Source: CAD feature listing. Evaluate the final solid. Frame: model axes, mm. A direction names the side the tool comes from. Give positions to 0.01 mm unless a question says otherwise; leave off trailing zeros. Order: outer loops, then holes, each group sorted by start corner. A loop starts at its lowest first (then second) coordinate and runs counter-clockwise, first axis right, second up. Notation, with made-up numbers: M -9,48 L 14,48 A20 ccw 14,60 Z; hole C 59.5,38 d6. An arc over 180 degrees is marked long. Use CSV: the item, a comma, the result in double quotes. Start each with the question number.
Item 1: Access query for faces 1 (the face through (0, 182, 23)), 2 (the face through (83.546, 357.97, 54.214)), 3 (the face through (152, 1.588, 38)). Directions: +Z, -Z, +X, -X, +Y, -Y. A direction counts if a zero-diameter tool reaches every point of the face in a straight line with its end or side. Return the directions, or none.
Item 2: First-contact query: pin 1 (6 mm diameter, centred on x = 40, y = 154.5, fed in from -Z); pin 2 (6 mm diameter, centred on x = 214, y = 196.5, fed in from +Z); pin 3 (1.3 mm diameter, centred on x = -2, y = 147, fed in from -Z); pin 4 (5 mm diameter, centred on y = 26.99, z = 52.39, fed in from -X). Flat tips, straight axial feed; report the tip coordinate or a pass-through.
Item 3: Section query A-A on y = 152.4. Return loops of the section in (x, z) (1 decimal).
Item 4: Pull-direction query (Z, two-part tool) for faces 4 (the face through (154, 358.775, 38)), 5 (the face through (152, 182, 0)), 6 (the face through (307.17, 141.382, 20.497)); classes: +Z half, -Z half, draft (parallel to the pull), parting line (faces both ways), or undercut.
Item 5: Ray query, probe 1 along X at (y, z) = (108, 60.5) (1 decimal); probe 2 along Y at (x, z) = (225.5, 13.5) (1 decimal); probe 3 along X at (y, z) = (183, 55) (1 decimal). Return the intervals inside material, ascending. Write a range as from..to.
Item 6: Section query C-C on x = 162.5. Return loops of the section in (y, z) (1 decimal), and give its area (3 significant figures).
Item 7: Section query D-D on x = 88.9. Count the separate pieces of the cut face and the enclosed holes in it, and give its area (3 significant figures).
Item 8: Section query B-B on z = 19.05. Return loops of the section in (x, y) (1 decimal), and give its area (3 significant figures).
Autodesk Inventor part; units mm, degrees
ref_plane "YZ Plane" through (0, 0, 0) normal (1, 0, 0) x (0, 1, 0)
ref_plane "XZ Plane" through (0, 0, 0) normal (0, 1, 0) x (-1, 0, 0)
ref_plane "XY Plane" through (0, 0, 0) normal (0, 0, 1) x (1, 0, 0)
sketch "Sketch1" plane through (0, 0, 0) normal (0, 0, 1) x (1, 0, 0)
  line L0 (0, 0) -> (307.975, 0)
  line L1 (307.975, 0) -> (307.975, 358.775)
  line L2 (307.975, 358.775) -> (0, 358.775)
  line L3 (0, 358.775) -> (0, 0)
  dimension "d0" = 307.975
  dimension "d1" = 358.775
extrude "Extrusion1" add sketch "Sketch1" along normal blind 76.2
shell "Shell1" thickness 1.5875 removed faces 1 at (205.3167, 119.5917, 76.2)
sketch "Sketch2" plane through (0, 358.775, 0) normal (0, 1, 0) x (1, 0, 0)
  line L0 (0, -76.2) -> (0, -60.325) construction
  line L1 (0, -60.325) -> (-3.175, -60.325) construction
  arc A0 (-2.3813, -58.7375) -> (-0.7938, -60.325) centre (-2.3813, -60.325) ccw
  line L2 (0, -60.325) -> (-0.7938, -60.325)
  line L3 (-0.7938, -58.7375) -> (-0.7938, -47.625)
  line L4 (-0.7938, -47.625) -> (0, -47.625)
  line L5 (0, -47.625) -> (0, -60.325)
  line L6 (-2.3813, -58.7375) -> (-0.7938, -58.7375)
  point P0 (0, 0)
  dimension "d10" = 15.875
  dimension "d11" = 3.175
  dimension "d12" = 3.175
  dimension "d13" = 12.7
extrude "Extrusion2" add sketch "Sketch2" against normal up to surface (358.775 mm away)
sketch "Sketch3" plane through (307.975, 0, 0) normal (1, 0, 0) x (0, 0, -1)
  line L0 (0, 358.775) -> (0, 0) construction
  line L1 (0, 0) -> (-19.05, 0) construction
  line L2 (-19.05, 0) -> (-19.05, 152.4) construction
  line L3 (-19.05, 152.4) -> (0, 152.4) construction
  line L4 (0, 152.4) -> (0, 0) construction
  dimension "d14" = 19.05
  dimension "d15" = 152.4
hole "Hole1" at (307.975, 152.4, 19.05) direction (-1, 0, 0) diameter 22.225 depth 25.4 tip angle 118
sketch "Sketch4" plane through (307.975, 0, 0) normal (1, 0, 0) x (0, 0, -1)
  line L0 (-1.5875, 357.1875) -> (-1.5875, 1.5875) construction
  line L1 (-1.5875, 1.5875) -> (-1.5875, 26.9875) construction
  line L2 (-1.5875, 26.9875) -> (-33.3375, 26.9875) construction
  line L3 (-1.5875, 26.9875) -> (-52.3875, 26.9875) construction
  point P0 (0, 0)
  dimension "d23" = 25.4
  dimension "d24" = 31.75
  dimension "d25" = 50.8
hole "Hole2" at (307.975, 26.9875, 52.3875) at (307.975, 26.9875, 33.3375) direction (-1, 0, 0) diameter 6.35 depth 25.4 tip angle 118
sketch "Sketch5" plane through (0, 358.775, 0) normal (0, 1, 0) x (1, 0, 0)
  line L0 (0, 0) -> (307.975, 0)
  line L1 (0, 0) -> (98.425, 0)
  line L2 (98.425, 0) -> (98.425, -22.225)
  dimension "d33" = 98.425
  dimension "d34" = 22.225
hole "Hole3" at (98.425, 358.775, 22.225) direction (0, -1, 0) diameter 28.575 depth 25.4 tip angle 118
sketch "Sketch6" plane through (0, 358.775, 0) normal (0, 1, 0) x (1, 0, 0)
  line L0 (0, -76.2) -> (307.975, -76.2) construction
  line L1 (0, -76.2) -> (88.9, -76.2) construction
  line L2 (88.9, -76.2) -> (88.9, -50.8) construction
  line L3 (88.9, -50.8) -> (0, -50.8) construction
  line L4 (0, -50.8) -> (0, -76.2) construction
  point P0 (0, 0)
  dimension "d42" = 88.9
  dimension "d43" = 25.4
hole "Hole4" at (88.9, 358.775, 50.8) direction (0, -1, 0) diameter 12.7 depth 25.4 tip angle 118
properties part number "case" material "Steel"
Verdict:
1,face 1,"-Z, -X, +Y, -Y"
1,face 2,"+Y"
1,face 3,"+Z"
2,pin 1,"z = 0"
2,pin 2,"z = 1.59"
2,pin 3,"z = 58.74"
2,pin 4,"x = -0.79"
3,outline,"M -2.4,58.7 L -0.8,58.7 L -0.8,47.6 L 0,47.6 L 0,0 L 308,0 L 308,7.9 L 306.4,7.9 L 306.4,1.6 L 1.6,1.6 L 1.6,76.2 L 0,76.2 L 0,60.3 L -0.8,60.3 A1.6 ccw long Z; M 306.4,30.2 L 308,30.2 L 308,76.2 L 306.4,76.2 Z"
4,face 4,"draft"
4,face 5,"-Z half"
4,face 6,"undercut"
5,probe 1,"-4..-0.8, 0..1.6, 306.4..308"
5,probe 2,"0..1.6, 357.2..358.8"
5,probe 3,"-0.8..1.6, 306.4..308"
6,outline,"M 0,0 L 358.8,0 L 358.8,76.2 L 357.2,76.2 L 357.2,1.6 L 1.6,1.6 L 1.6,76.2 L 0,76.2 Z"
6,area,"806 mm2"
7,separate pieces,"3"
7,enclosed holes,"0"
7,area,"752 mm2"
8,outline,"M 0,0 L 308,0 L 308,141.3 L 306.4,141.3 L 306.4,1.6 L 1.6,1.6 L 1.6,357.2 L 84.5,357.2 L 84.5,358.8 L 0,358.8 Z; M 112.4,357.2 L 306.4,357.2 L 306.4,163.5 L 308,163.5 L 308,358.8 L 112.4,358.8 Z"
8,area,"2,030 mm2"
